CAD build for the part. Positions are in the model's coordinates, mm. Coordinates: 2 decimals unless noted, no trailing zeros. Order: outer loops, then holes, each group sorted by start corner. A loop starts at its lowest first (then second) coordinate and runs counter-clockwise, first axis right, second up. Notation, with made-up numbers: M 61.5,15 L 92.5,15 A35 ccw 92.5,54 Z; hole C 13,2.5 d11. An arc over 180 degrees is marked long. Write item = value, one per line. Start each with the question number.
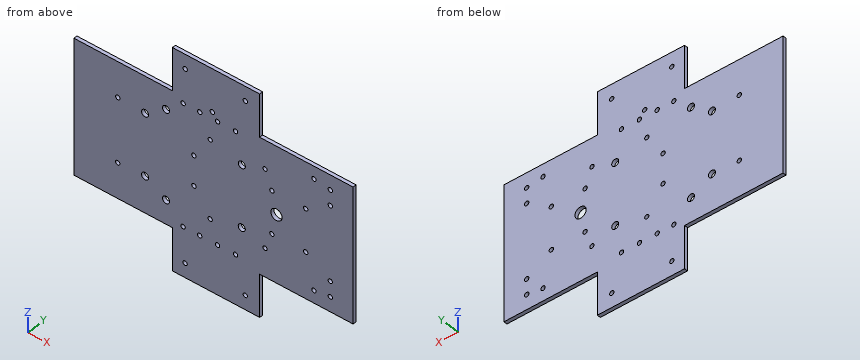
```python
from build123d import *

# Parameters (mm, degrees)
SKETCH_1_R      = 1.5
SKETCH_1_R_2    = 4
SKETCH_1_R_3    = 2.5
SKETCH_1_R_4    = 1.55
EXTRUDE_1_DEPTH = 2.5


with BuildPart() as part:
    # 草图1 → 凸台-拉伸1 (new body)
    with BuildSketch(Plane(origin=(0, 0, 0), x_dir=(1, 0, 0), z_dir=(0, 1, 0))):
        Polygon((0, 95), (70, 95), (70, 125), (132, 125), (132, 95), (198.395701384, 95), (198.395701384, 0), (132, 0), (132, -30), (70, -30), (70, 0), (0, 0), align=None)
        with Locations(Location((96.855482095, 20, 0), (0, 0, 270))):
            Circle(SKETCH_1_R, mode=Mode.SUBTRACT)
        with Locations(Location((135.855482095, 20, 0), (0, 0, 270))):
            Circle(SKETCH_1_R, mode=Mode.SUBTRACT)
        with Locations(Location((96.855482095, 75, 0), (0, 0, 270))):
            Circle(SKETCH_1_R, mode=Mode.SUBTRACT)
        with Locations(Location((135.855482095, 75, 0), (0, 0, 270))):
            Circle(SKETCH_1_R, mode=Mode.SUBTRACT)
        with Locations(Location((143.91825516, 47.568677235, 0), (0, 0, 270))):
            Circle(SKETCH_1_R_2, mode=Mode.SUBTRACT)
        with Locations(Location((65.477875917, 15.309382071, 0), (0, 0, 270))):
            Circle(SKETCH_1_R_3, mode=Mode.SUBTRACT)
        with Locations(Location((65.477875917, 78.060864371, 0), (0, 0, 270))):
            Circle(SKETCH_1_R_3, mode=Mode.SUBTRACT)
        with Locations(Location((50.549464097, 69.348606616, 0), (0, 0, 270))):
            Circle(SKETCH_1_R_3, mode=Mode.SUBTRACT)
        with Locations(Location((119.28195754, 69.348606616, 0), (0, 0, 270))):
            Circle(SKETCH_1_R_3, mode=Mode.SUBTRACT)
        with Locations(Location((85.282184512, 58, 0), (0, 0, 270))):
            Circle(SKETCH_1_R_4, mode=Mode.SUBTRACT)
        with Locations(Location((85.282184512, 37, 0), (0, 0, 270))):
            Circle(SKETCH_1_R_4, mode=Mode.SUBTRACT)
        with Locations(Location((119.302755352, 25.765245087, 0), (0, 0, 270))):
            Circle(SKETCH_1_R_3, mode=Mode.SUBTRACT)
        with Locations(Location((50.570293212, 25.699647342, 0), (0, 0, 270))):
            Circle(SKETCH_1_R_3, mode=Mode.SUBTRACT)
        with Locations(Location((140.705086193, 62.572870277, 0), (0, 0, 270))):
            Circle(SKETCH_1_R_4, mode=Mode.SUBTRACT)
        with Locations(Location((164.705086193, 62.572870277, 0), (0, 0, 270))):
            Circle(SKETCH_1_R_4, mode=Mode.SUBTRACT)
        with Locations(Location((140.705086193, 32.572870277, 0), (0, 0, 270))):
            Circle(SKETCH_1_R_4, mode=Mode.SUBTRACT)
        with Locations(Location((164.705086193, 32.572870277, 0), (0, 0, 270))):
            Circle(SKETCH_1_R_4, mode=Mode.SUBTRACT)
        with Locations(Location((79.074216313, -19.848364995, 0), (0, 0, 270))):
            Circle(SKETCH_1_R_4, mode=Mode.SUBTRACT)
        with Locations(Location((121.803446989, -19.848364995, 0), (0, 0, 270))):
            Circle(SKETCH_1_R_4, mode=Mode.SUBTRACT)
        with Locations(Location((79.009903556, 114.923802126, 0), (0, 0, 270))):
            Circle(SKETCH_1_R_4, mode=Mode.SUBTRACT)
        with Locations(Location((121.739114772, 114.964582564, 0), (0, 0, 270))):
            Circle(SKETCH_1_R_4, mode=Mode.SUBTRACT)
        with Locations(Location((31.137813249, 24.825739094, 0), (0, 0, 270))):
            Circle(SKETCH_1_R_4, mode=Mode.SUBTRACT)
        with Locations(Location((31.116158933, 70.203968261, 0), (0, 0, 270))):
            Circle(SKETCH_1_R_4, mode=Mode.SUBTRACT)
        with Locations(Location((77.583731052, 90.347159974, 0), (0, 0, 270))):
            Circle(SKETCH_1_R_4, mode=Mode.SUBTRACT)
        with Locations(Location((89.406896358, 90.347159974, 0), (0, 0, 270))):
            Circle(SKETCH_1_R_4, mode=Mode.SUBTRACT)
        with Locations(Location((98.355349988, 0, 0), (0, 0, 270))):
            Circle(SKETCH_1_R_4, mode=Mode.SUBTRACT)
        with Locations(Location((102.054410992, 90.347159974, 0), (0, 0, 270))):
            Circle(SKETCH_1_R_4, mode=Mode.SUBTRACT)
        with Locations(Location((114.840909304, 90.347159974, 0), (0, 0, 270))):
            Circle(SKETCH_1_R_4, mode=Mode.SUBTRACT)
        with Locations(Location((114.88174999, 4.762462791, 0), (0, 0, 270))):
            Circle(SKETCH_1_R_4, mode=Mode.SUBTRACT)
        with Locations(Location((102.095257502, 4.750259459, 0), (0, 0, 270))):
            Circle(SKETCH_1_R_4, mode=Mode.SUBTRACT)
        with Locations(Location((89.447748628, 4.738188772, 0), (0, 0, 270))):
            Circle(SKETCH_1_R_4, mode=Mode.SUBTRACT)
        with Locations(Location((77.624588706, 4.726904837, 0), (0, 0, 270))):
            Circle(SKETCH_1_R_4, mode=Mode.SUBTRACT)
        with Locations(Location((170.569167864, 86.187416053, 0), (0, 0, 270))):
            Circle(SKETCH_1_R_4, mode=Mode.SUBTRACT)
        with Locations(Location((182.194893719, 84.546137109, 0), (0, 0, 270))):
            Circle(SKETCH_1_R_4, mode=Mode.SUBTRACT)
        with Locations(Location((182.194893719, 73.741050727, 0), (0, 0, 270))):
            Circle(SKETCH_1_R_4, mode=Mode.SUBTRACT)
        with Locations(Location((182.194893719, 21.258949273, 0), (0, 0, 270))):
            Circle(SKETCH_1_R_4, mode=Mode.SUBTRACT)
        with Locations(Location((182.194893719, 10.453862891, 0), (0, 0, 270))):
            Circle(SKETCH_1_R_4, mode=Mode.SUBTRACT)
        with Locations(Location((170.569167864, 8.812583947, 0), (0, 0, 270))):
            Circle(SKETCH_1_R_4, mode=Mode.SUBTRACT)
    extrude(amount=EXTRUDE_1_DEPTH)


solid = part.part
```
1. Probe L1, parallel to X at y = 0.9, z = -74; L2, parallel to Z at x = 169.5, y = 1.45; L3, parallel to X at y = 0.3, z = -47. List the from-to ranges inside material, lowest first.
2. Slice it at C-C (y = 0.8). Give the number of separate pieces and of enclosed holes in the cut face, plus the area to 3 significant figures.
3. Slice it at A-A (z = -46.5). Write the cut outline in (x, y), plus the area to 3 significant figures.
4. Slice it at B-B (z = 11). Write the cut outline in (x, y), plus the area to 3 significant figures.
5. Slice it at D-D (x = 42). Write the cut outline in (y, z), plus the area to 4 significant figures.
6. Flat gauge pins, fed straight in: pin 1 (1 mm diameter, centred on y = 1.5, z = -98, fed in from +X); pin 2 (5 mm diameter, centred on x = 164.71, z = -62.57, fed in from +Y); pin 3 (1.5 mm diameter, centred on x = 46, y = 1, fed in from +Z). Where does each tip first touch, or does it go through?
Calculated:
q1.L1 = 0 to 95.74, 97.97 to 134.74, 136.97 to 180.67, 183.72 to 198.4
q1.L2 = -95 to -87.31, -85.07 to -9.93, -7.69 to 0
q1.L3 = 0 to 139.96, 147.88 to 198.4
q2.separate_pieces = 1
q2.enclosed_holes = 38
q2.area = 22,200 mm²
q3.outline = M 0,0 L 140.06,0 L 140.06,2.5 L 0,2.5 Z; M 147.77,0 L 198.4,0 L 198.4,2.5 L 147.77,2.5 Z
q3.area = 477 mm²
q4.outline = M 70,0 L 132,0 L 132,2.5 L 70,2.5 Z
q4.area = 155 mm²
q5.outline = M 0,-95 L 2.5,-95 L 2.5,0 L 0,0 Z
q5.area = 237.5 mm²
q6.pin_1 = 132
q6.pin_2 = 2.5
q6.pin_3 = 0
